Can you work these out from the model? Positions are in its coordinate system, mm. A direction names the side the tool comes from. Give positions to 0.01 mm unless a question says otherwise; leave off trailing zeros. Order: outer loops, then holes, each group sorted by start corner. A loop starts at its lowest first (then second) coordinate and runs counter-clockwise, first axis right, second up. Notation, with made-up numbers: M 39,86 L 98,86 A17 ccw 98,108 Z; hole C 42,13.5 d6. An arc over 180 degrees is marked long. Use one line per item in the form item = value. Start each with the question number.
1. I want a section at A-A, the plane z = -35. List the corners of the cut face in (x, y) for me.
2. I need wall thicknesses on L1, parallel to Z at x = 0, y = 2.1; L2, parallel to Y at x = 1.5, z = -18; L3, parallel to X at y = -2.75, z = -9. Which ranges of each line are inside material? Lowest first, please.
3. Will these pins go through, and if not, where does the flat tip stop? P1, Ø2, axis at x = 23, z = -10.5, coming from the -Y side; P2, Ø4, axis at y = -0.5, z = -7, coming from the +X side; P3, Ø3.5, axis at y = -6, z = -22, coming from the +X side; P4, Ø6, axis at x = 14.5, y = -3.5, coming from the -Z side.
4. We'd pull the mould along X, two halves only. Please class faces 6 (the face through (1.216, 1.479, -1.115)), 7 (the face through (20.43, -6.08, -4.6)), 8 (the face through (-0.89, 1.48, -36.39)), 9 (the face through (13, 3, -17)): +X half, -X half, draft (parallel to the pull), parting line (faces both ways), or undercut.
5. For faces 1 (the face through (4.57, -6.08, -30.4)), 2 (the face through (4.6, -6.08, -4.57)), 3 (the face through (4, -6, -18)), 4 (the face through (20.4, -6.08, -30.43)), 5 (the face through (13, -6, -31)), which set-ups out of +Z, -Z, +X, -X, +Y, -Y let a thin tool reach every point of the face, with its end or its side?
6. I want a section at B-B, the plane x = 17. List the corners of the cut face in (y, z) for me.
7. I want a section at D-D, the plane x = 0. List the corners of the cut face in (y, z) for me.
8. I want a section at C-C, the plane y = 1.5. List the corners of the cut face in (x, z) for me.
Autodesk Inventor part; units mm, degrees
ref_plane "YZ Plane" through (0, 0, 0) normal (1, 0, 0) x (0, 1, 0)
ref_plane "XZ Plane" through (0, 0, 0) normal (0, 1, 0) x (-1, 0, 0)
ref_plane "XY Plane" through (0, 0, 0) normal (0, 0, 1) x (1, 0, 0)
sketch "Sketch1" plane through (0, 0, 0) normal (0, 1, 0) x (-1, 0, 0)
  circle A0 centre (0, 0) radius 1.65
  circle A1 centre (0, -35) radius 1.65
  circle A2 centre (-25, 0) radius 1.65
  circle A3 centre (-25, -35) radius 1.65
  line L0 (0, 0) -> (-25, 0) construction
  line L1 (-25, 0) -> (-25, -35) construction
  line L2 (-25, -35) -> (0, -35) construction
  line L3 (0, -35) -> (0, 0) construction
  line L4 (4, 4) -> (-29, 4)
  line L5 (-29, 4) -> (-29, -39)
  line L6 (-29, -39) -> (4, -39)
  line L7 (4, -39) -> (4, 4)
  dimension "d1" = 3.3
  dimension "d2" = 3.3
  dimension "d4" = 3.3
  dimension "d5" = 3.3
  dimension "d6" = 35
  dimension "d7" = 25
  dimension "d8" = 4
extrude "Extrusion1" add sketch "Sketch1" along normal blind 3
sketch "Sketch2" plane through (0, 0, 0) normal (0, -1, 0) x (1, 0, 0)
  circle A0 centre (25, -35) radius 1.65 construction
  circle A1 centre (25, 0) radius 1.65 construction
  circle A2 centre (0, -35) radius 1.65 construction
  circle A3 centre (0, 0) radius 1.65 construction
  line L0 (29, -39) -> (-4, -39)
  line L1 (-4, -39) -> (-4, 4)
  line L2 (-4, 4) -> (29, 4)
  line L3 (29, 4) -> (29, -39)
  line L4 (21, -31) -> (4, -31)
  line L5 (4, -31) -> (4, -4)
  line L6 (4, -4) -> (21, -4)
  line L7 (21, -4) -> (21, -31)
  dimension "d11" = 8
extrude "Extrusion2" add sketch "Sketch2" along normal blind 12 contours L4 L5 L6 L7
fillet "Fillet1" radius 2 8 edges at (29, 1.5, 4) (-4, 1.5, 4) (-4, 1.5, -39) (29, 1.5, -39) (21, -6, -4) (4, -6, -4) (4, -6, -31) (21, -6, -31)
properties part number "gravity-pcb-mount"
Check result:
q1.outline = M -4,0 L -1.65,0 L -1.65,3 L -4,3 Z; M 1.65,0 L 23.35,0 L 23.35,3 L 1.65,3 Z; M 26.65,0 L 29,0 L 29,3 L 26.65,3 Z
q2.L1 = -39 to -36.65, -33.35 to -1.65, 1.65 to 4
q2.L2 = 0 to 3
q2.L3 = 4 to 21
q3.P1 = 0
q3.P2 = 29
q3.P3 = 21
q3.P4 = -31
q4.face_6 = undercut
q4.face_7 = +X half
q4.face_8 = undercut
q4.face_9 = draft
q5.face_1 = -Z, -X, -Y
q5.face_2 = +Z, -X, -Y
q5.face_3 = +Z, -Z, -X, -Y
q5.face_4 = -Z, +X, -Y
q5.face_5 = -Z, +X, -X, -Y
q6.outline = M -12,-31 L 0,-31 L 0,-39 L 3,-39 L 3,4 L 0,4 L 0,-4 L -12,-4 Z
q7.outline = M 0,-39 L 3,-39 L 3,-36.65 L 0,-36.65 Z; M 0,-33.35 L 3,-33.35 L 3,-1.65 L 0,-1.65 Z; M 0,1.65 L 3,1.65 L 3,4 L 0,4 Z
q8.outline = M -4,-37 A2 ccw -2,-39 L 27,-39 A2 ccw 29,-37 L 29,2 A2 ccw 27,4 L -2,4 A2 ccw -4,2 Z; hole C 0,-35 d3.3; hole C 0,0 d3.3; hole C 25,-35 d3.3; hole C 25,0 d3.3
